Can you work these out from the model? Positions are in its coordinate system, mm. Give positions to 0.01 mm unless a question says otherwise; leave off trailing zeros. Write each loop counter-clockwise with the first axis right and the second up, starting at its lowest first coordinate (ties: lowest second). Pieces come first, ordered by that corner, then holes.
```python
from build123d import *

# Parameters (mm, degrees)
SKETCH2_W           = 806
SKETCH2_H           = 605
BOSS_EXTRUDE1_DEPTH = 19
SKETCH4_W           = 25
SKETCH4_H           = 25
BOSS_EXTRUDE3_DEPTH = 710
FILLET2_R           = 40
FILLET3_R           = 40
FILLET4_R           = 40


with BuildPart() as part:
    # Sketch2 → Boss-Extrude1 (new body)
    with BuildSketch(Plane(origin=(0, 0, 0), x_dir=(1, 0, 0), z_dir=(0, 1, 0))):
        Rectangle(SKETCH2_W, SKETCH2_H)
    extrude(amount=BOSS_EXTRUDE1_DEPTH)

    # Sketch4 → Boss-Extrude3 (add)
    with BuildSketch(Plane.XZ):
        with Locations((-360.678585118, 265)):
            Rectangle(SKETCH4_W, SKETCH4_H)
        with Locations((365.5, 265)):
            Rectangle(SKETCH4_W, SKETCH4_H)
        with Locations((365.5, -265)):
            Rectangle(SKETCH4_W, SKETCH4_H)
        with Locations((-365.5, -265)):
            Rectangle(SKETCH4_W, SKETCH4_H)
    extrude(amount=BOSS_EXTRUDE3_DEPTH)

    # Fillet2
    fillet2_edges = [part.edges().sort_by_distance(p)[0] for p in [
        (403, 9.5, 302.5),
    ]]
    fillet(fillet2_edges, radius=FILLET2_R)

    # Fillet3
    fillet3_edges = [part.edges().sort_by_distance(p)[0] for p in [
        (-403, 9.5, 302.5),
    ]]
    fillet(fillet3_edges, radius=FILLET3_R)

    # Fillet4
    fillet4_edges = [part.edges().sort_by_distance(p)[0] for p in [
        (-403, 9.5, -302.5),
        (403, 9.5, -302.5),
    ]]
    fillet(fillet4_edges, radius=FILLET4_R)


solid = part.part
```
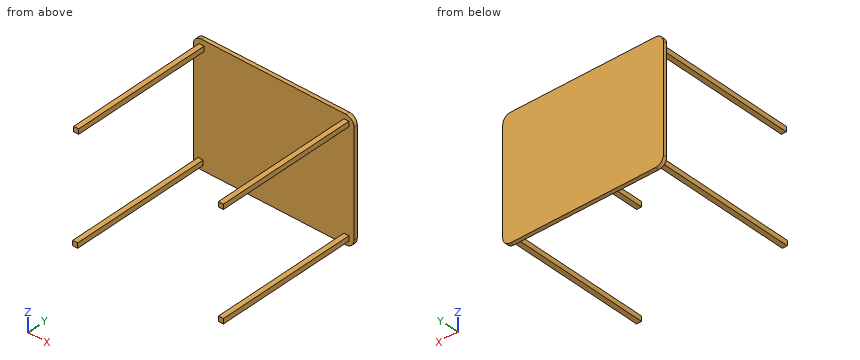
1) Suppose I cut it at A-A on y = -183. Write out the boundary of the cut face in (x, z), plus the area to 3 significant figures.
Values follow:
outline: (-378, -277.5) - (-353, -277.5) - (-353, -252.5) - (-378, -252.5) - close; (-373.18, 252.5) - (-348.18, 252.5) - (-348.18, 277.5) - (-373.18, 277.5) - close; (353, -277.5) - (378, -277.5) - (378, -252.5) - (353, -252.5) - close; (353, 252.5) - (378, 252.5) - (378, 277.5) - (353, 277.5) - close
area: 2,500 mm2
2) For pin 1 Ø10 at (x, z) = (188.5, 183) entering from -Y; pin 2 Ø7.5 at (y, z) = (-494.5, -271) entering from +X; pin 3 Ø20 at (x, y) = (-371, -365) entering from +Z, each with a flat end and sliding along its axis, tell me the tip position at first contact or that it passes through.
Values follow:
pin 1: stops at y = 0
pin 2: stops at x = 378
pin 3: stops at z = 277.5
3) Please list where these lines run through material, in increasing order: L1, parallel to Y at x = -271.5, z = -258.5; L2, parallel to X at y = -436.5, z = -271.
Values follow:
L1: y = 0 to 19
L2: x = -378 to -353, 353 to 378
4) Suppose I cut it at B-B on z = -175. Write out the boundary of the cut face in (x, y), plus the area to 3 significant figures.
Values follow:
outline: (-403, 0) - (403, 0) - (403, 19) - (-403, 19) - close
area: 15,300 mm2
5) Suppose I cut it at C-C on x = 159. Write out the boundary of the cut face in (y, z).
Values follow:
outline: (0, -302.5) - (19, -302.5) - (19, 302.5) - (0, 302.5) - close
